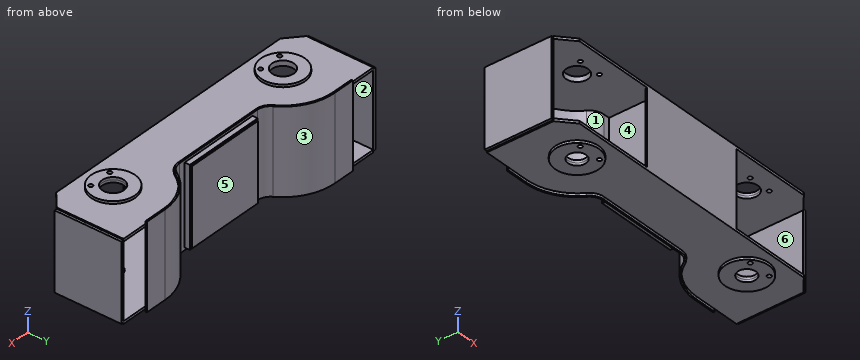
```python
from build123d import *

# Parameters (mm, degrees)
SKETCH_1_R          = 35
SKETCH_1_R_2        = 8
EXTRUDE_1_DEPTH     = 310
SKETCH_2_W          = 1176
SKETCH_2_H          = 290
CUT_EXTRUDE_1_DEPTH = 735.294218961
EXTRUDE_2_DEPTH     = 330
SKETCH_4_R          = 42.5
CUT_EXTRUDE_2_DEPTH = 10
SKETCH_5_R          = 85
SKETCH_5_R_2        = 42.5
SKETCH_5_R_3        = 8
EXTRUDE_3_DEPTH     = 10
SKETCH_6_R          = 85
SKETCH_6_R_2        = 8
SKETCH_6_R_3        = 35
EXTRUDE_4_DEPTH     = 10
SKETCH_7_W          = 10
SKETCH_7_H          = 290
EXTRUDE_5_DEPTH     = 184
SKETCH_8_W          = 420
SKETCH_8_H          = 290
EXTRUDE_6_DEPTH     = 6
SKETCH_9_W          = 10
SKETCH_9_H          = 300
EXTRUDE_7_DEPTH     = 260
SKETCH_10_W         = 320
SKETCH_10_H         = 310
EXTRUDE_8_DEPTH     = 20
SKETCH_11_W         = 310
SKETCH_11_H         = 300
EXTRUDE_9_DEPTH     = 5


with BuildPart() as part:
    # Sketch 1 → Extrude 1 (new body)
    with BuildSketch(Plane.XY):
        with BuildLine():
            Line((0, 0), (0, 190))
            Line((0, 190), (184, 190))
            ThreePointArc((184, 190), (211.540328216, 197.240074634), (231.959441014, 217.088202795))
            ThreePointArc((231.959441014, 217.088202795), (303.504043203, 286.632185805), (400, 312))
            Line((400, 312), (588, 312))
            Line((588, 312), (588, 52))
            Line((588, 52), (528, 0))
            Line((528, 0), (0, 0))
        make_face()
        with Locations((400, 116)):
            Circle(SKETCH_1_R, mode=Mode.SUBTRACT)
        with Locations((355, 66)):
            Circle(SKETCH_1_R_2, mode=Mode.SUBTRACT)
        with Locations((445, 66)):
            Circle(SKETCH_1_R_2, mode=Mode.SUBTRACT)
    extrude_1 = extrude(amount=EXTRUDE_1_DEPTH)

    # Mirror 1: Extrude 1 across plane
    add(extrude_1.mirror(Plane(origin=(0, 0, 0), x_dir=(0, 0, 1), z_dir=(1, 0, 0))))

    # Sketch 2 → Cut-Extrude 1 (cut, through all)
    with BuildSketch(Plane(origin=(0, 0, 0), x_dir=(-1, 0, 0), z_dir=(0, -1, 0))):
        with Locations((0, -155)):
            Rectangle(SKETCH_2_W, SKETCH_2_H)
    extrude(amount=-CUT_EXTRUDE_1_DEPTH, mode=Mode.SUBTRACT)


with BuildPart() as cut_extrude_1_piece_1:
    # of the separate pieces the step leaves, piece 1, a body of its own (cut_extrude_1_pieces)
    add(part.part.solids().sort_by_distance((184, 190, 0))[0])



with BuildPart() as cut_extrude_1_piece_2:
    # of the separate pieces the step leaves, piece 2, a body of its own (cut_extrude_1_pieces)
    add(part.part.solids().sort_by_distance((184, 190, 300))[0])

    # Sketch 4 → Cut-Extrude 2 (cut)
    with BuildSketch(Plane.XY.offset(310)):
        with Locations((-400, 116)):
            Circle(SKETCH_4_R)
        with Locations((400, 116)):
            Circle(SKETCH_4_R)
    extrude(amount=-CUT_EXTRUDE_2_DEPTH, mode=Mode.SUBTRACT)


with BuildPart() as body_3:
    # Sketch 3 → Extrude 2 (new body)
    with BuildSketch(Plane.XY.offset(320)):
        with BuildLine():
            Line((-184, 190), (184, 190))
            ThreePointArc((184, 190), (211.540328216, 197.240074634), (231.959441014, 217.088202795))
            ThreePointArc((231.959441014, 217.088202795), (303.504043203, 286.632185805), (400, 312))
            Line((400, 312), (485, 312))
            Line((485, 312), (485, 318))
            Line((485, 318), (400, 318))
            ThreePointArc((400, 318), (300.553293751, 291.856463523), (226.820929477, 220.185895353))
            ThreePointArc((226.820929477, 220.185895353), (208.589578764, 202.464352351), (184, 196))
            Line((184, 196), (-184, 196))
            ThreePointArc((-184, 196), (-208.589578764, 202.464352351), (-226.820929477, 220.185895353))
            ThreePointArc((-226.820929477, 220.185895353), (-300.553293751, 291.856463523), (-400, 318))
            Line((-400, 318), (-485, 318))
            Line((-485, 318), (-485, 312))
            Line((-485, 312), (-400, 312))
            ThreePointArc((-400, 312), (-303.504043203, 286.632185805), (-231.959441014, 217.088202795))
            ThreePointArc((-231.959441014, 217.088202795), (-211.540328216, 197.240074634), (-184, 190))
        make_face()
    extrude(amount=-EXTRUDE_2_DEPTH)


    add(cut_extrude_1_piece_2.part)  # Extrude 3 merges Cut-Extrude 1 piece 2
    # Sketch 5 → Extrude 3 (add)
    # profile 1 of 2: a face of its own
    with BuildSketch(Plane.XY.offset(310)):
        with Locations((-400, 116)):
            Circle(SKETCH_5_R)
        with Locations((-400, 116)):
            Circle(SKETCH_5_R_2, mode=Mode.SUBTRACT)
        with Locations(Location((-355, 66, 0), (0, 0, 180))):
            Circle(SKETCH_5_R_3, mode=Mode.SUBTRACT)
        with Locations(Location((-445, 66, 0), (0, 0, 180))):
            Circle(SKETCH_5_R_3, mode=Mode.SUBTRACT)
    # profile 2 of 2: a face of its own
    with BuildSketch(Plane.XY.offset(310)):
        with Locations((400, 116)):
            Circle(SKETCH_5_R)
        with Locations(Location((355, 66, 0), (0, 0, 180))):
            Circle(SKETCH_5_R_3, mode=Mode.SUBTRACT)
        with Locations(Location((445, 66, 0), (0, 0, 180))):
            Circle(SKETCH_5_R_3, mode=Mode.SUBTRACT)
        with Locations((400, 116)):
            Circle(SKETCH_5_R_2, mode=Mode.SUBTRACT)
    extrude(amount=EXTRUDE_3_DEPTH)


with BuildPart() as cut_extrude_1_piece_1_1:
    add(cut_extrude_1_piece_1.part)

    add(body_3.part)  # Extrude 4 merges body 3
    # Sketch 6 → Extrude 4 (add)
    # profile 1 of 2: a face of its own
    with BuildSketch(Plane(origin=(0, 0, 0), x_dir=(-1, 0, 0), z_dir=(0, 0, -1))):
        with Locations(Location((-400, 116, 0), (0, 0, 180))):
            Circle(SKETCH_6_R)
        with Locations((-355, 66)):
            Circle(SKETCH_6_R_2, mode=Mode.SUBTRACT)
        with Locations((-445, 66)):
            Circle(SKETCH_6_R_2, mode=Mode.SUBTRACT)
        with Locations((-400, 116)):
            Circle(SKETCH_6_R_3, mode=Mode.SUBTRACT)
    # profile 2 of 2: a face of its own
    with BuildSketch(Plane(origin=(0, 0, 0), x_dir=(-1, 0, 0), z_dir=(0, 0, -1))):
        with Locations(Location((400, 116, 0), (0, 0, 180))):
            Circle(SKETCH_6_R)
        with Locations((445, 66)):
            Circle(SKETCH_6_R_2, mode=Mode.SUBTRACT)
        with Locations((355, 66)):
            Circle(SKETCH_6_R_2, mode=Mode.SUBTRACT)
        with Locations((400, 116)):
            Circle(SKETCH_6_R_3, mode=Mode.SUBTRACT)
    extrude(amount=EXTRUDE_4_DEPTH)

    # Sketch 7 → Extrude 5 (add)
    with BuildSketch(Plane(origin=(0, 190, 0), x_dir=(-1, 0, 0), z_dir=(0, -1, 0))):
        with Locations((-105, -155)):
            Rectangle(SKETCH_7_W, SKETCH_7_H)
        with Locations((-155, -155)):
            Rectangle(SKETCH_7_W, SKETCH_7_H)
        with Locations((105, -155)):
            Rectangle(SKETCH_7_W, SKETCH_7_H)
        with Locations((155, -155)):
            Rectangle(SKETCH_7_W, SKETCH_7_H)
    extrude(amount=EXTRUDE_5_DEPTH)

    # Sketch 8 → Extrude 6 (add)
    with BuildSketch(Plane.XZ):
        with Locations((0, 155)):
            Rectangle(SKETCH_8_W, SKETCH_8_H)
    extrude(amount=-EXTRUDE_6_DEPTH)

    # Sketch 9 → Extrude 7 (add)
    with BuildSketch(Plane(origin=(0, 312, 0), x_dir=(1, 0, 0), z_dir=(0, 1, 0))):
        with Locations((593, -155)):
            Rectangle(SKETCH_9_W, SKETCH_9_H)
        with Locations((-593, -155)):
            Rectangle(SKETCH_9_W, SKETCH_9_H)
    extrude(amount=-EXTRUDE_7_DEPTH)

    # Sketch 10 → Extrude 8 (add)
    with BuildSketch(Plane(origin=(0, 196, 0), x_dir=(1, 0, 0), z_dir=(0, 1, 0))):
        with Locations((0, -155)):
            Rectangle(SKETCH_10_W, SKETCH_10_H)
    extrude(amount=EXTRUDE_8_DEPTH)

    # Sketch 11 → Extrude 9 (add)
    with BuildSketch(Plane(origin=(0, 216, 0), x_dir=(1, 0, 0), z_dir=(0, 1, 0))):
        with Locations((0, -155)):
            Rectangle(SKETCH_11_W, SKETCH_11_H)
    extrude(amount=EXTRUDE_9_DEPTH)


solid = cut_extrude_1_piece_1_1.part
```
Could you check a few things on this model? Use its own coordinates, in mm. Face numbers are marked on the shaded views. A direction names the side the tool comes from. Round coordinates to 2 decimals unless told otherwise and drop trailing zeros. Order: outer loops, then holes, each group sorted by start corner. A loop starts at its lowest first (then second) coordinate and runs counter-clockwise, first axis right, second up. Notation, with made-up numbers: M 56.5,-21.75 L 79.5,-21.75 A15 ccw 79.5,1.25 Z; hole C 87,-26 d1. An arc over 180 degrees is marked long. One line per question, with ' | ' between items. Start each with the question number.
(1) For the marked faces 4, 5 and 6, which set-ups out of +Z, -Z, +X, -X, +Y, -Y let a thin tool reach every point of the face, with its end or its side?
(2) Please list where these lines run through material, in increasing order: line 1 along X through (y, z) = (66, 307); line 2 along X through (y, z) = (161, 24); line 3 along Z through (x, y) = (-98, 188.5).
(3) Suppose I cut it at B-B on z = 227. Count the separate pieces of the cut face and the enclosed holes in it, then the cut area to 3 significant figures.
(4) Thinking about a two-plate mould opening in Y: for the marked faces 1, 2 and 3, which applies, +Y half, -Y half, draft (parallel to the pull), parting line (faces both ways), or undercut?
(5) For P1, Ø12, axis at x = 133, y = 86, coming from the -Z side; P2, Ø2, axis at x = 255.5, y = 87, coming from the +Z side; P3, Ø11, axis at x = 594, y = 118.5, coming from the -Z side; P4, Ø13, axis at x = 355, y = 66, coming from the +Z side, each with a flat end and sliding along its axis, tell me the tip position at first contact or that it passes through.
(6) Suppose I cut it at A-A on x = 11.5. List the corners of the cut face in (y, z) for me.
Geometry results:
1) face 4: none | face 5: +Z, -Z, +Y | face 6: +Y, -Y
2) line 1: -588 to -453, -437 to -363, -347 to 347, 363 to 437, 453 to 588 | line 2: -598 to -588, -160 to -150, -110 to -100, 100 to 110, 150 to 160, 588 to 598 | line 3: 0 to 10, 300 to 310
3) separate pieces: 3 | enclosed holes: 3 | area: 29,400 mm²
4) face 1: undercut | face 2: draft | face 3: +Y half
5) P1: z = 0 | P2: z = 310 | P3: z = 5 | P4: through
6) outline: M 0,0 L 190,0 L 190,-10 L 196,-10 L 196,0 L 216,0 L 216,5 L 221,5 L 221,305 L 216,305 L 216,310 L 196,310 L 196,320 L 190,320 L 190,310 L 0,310 Z; hole M 6,10 L 190,10 L 190,300 L 6,300 Z
